Study the drawing (mm; zero at the part's minimum x, y, z) and answer. A direction names the side the tool comes from. Give positions to 0.01 mm unless a question says otherwise; leave off trailing zeros. Order: outer loops, then holes, each group sorted by start corner. A loop starts at its lowest first (then second) coordinate and runs counter-clockwise, first axis right, second up. Notation, with made-up numbers: (-11.75, -37) - (-6.75, -37) arc R23 ccw to (-6.75, -13) - close; hole circle Ø5 at (76, 15). An arc over 180 degrees is marked (long way). Return JSON: item names as keys, results as strings.
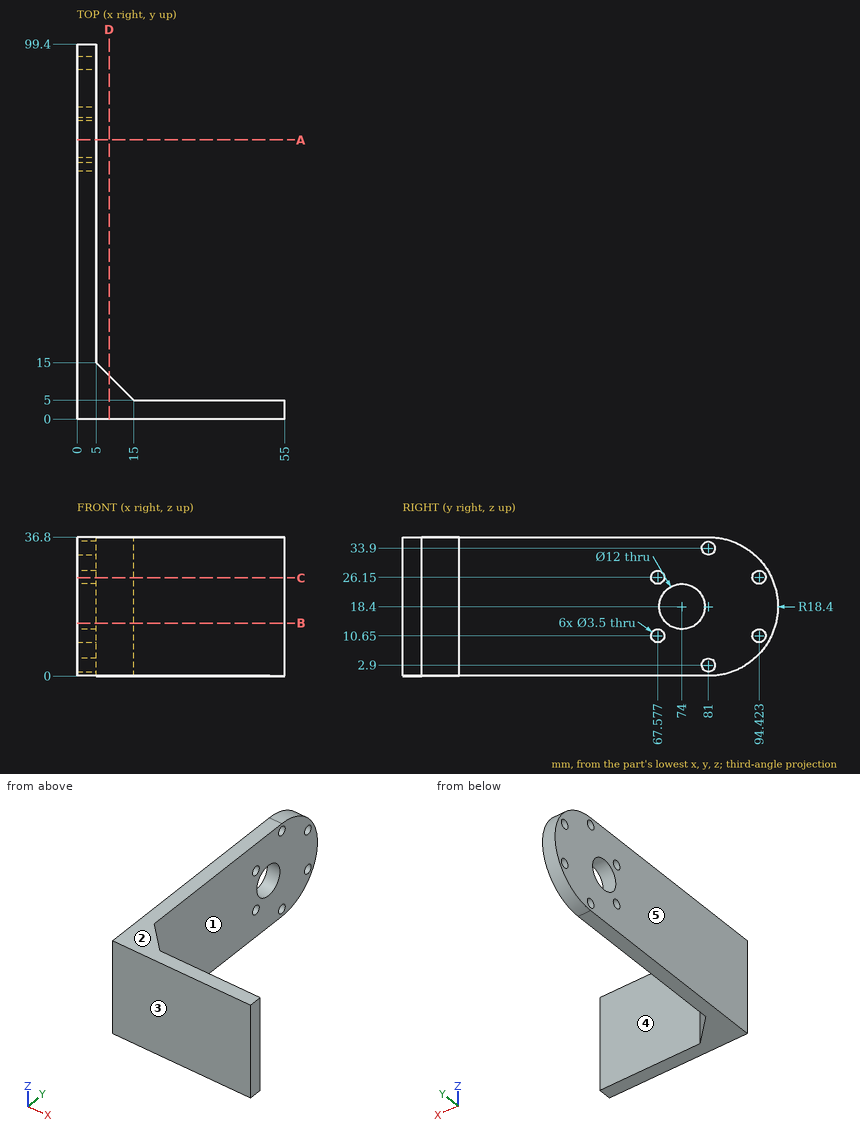
Q1. For the marked faces 1 and 2, determine the directions among +Z, -Z, +X, -X, +Y, -Y from which every point of the face is accessible in a straight line to the end or side of a thin tool.
Values:
{"face 1": "+Z, -Z, +X, +Y", "face 2": "+Z, +X, -X, +Y, -Y"}
Q2. A cutting plane is placed at D-D (x = 8.5). Write down the section's boundary in (y, z).
Values:
{"outline": "(0, 0) - (11.5, 0) - (11.5, 36.8) - (0, 36.8) - close"}
Q3. Determine the mould class of the marked faces 3, 4 and 5 for opening direction Y: released by +Y, released by -Y, zero draft, split by the parting line, or undercut.
Values:
{"face 3": "released by -Y", "face 4": "released by +Y", "face 5": "zero draft"}
Q4. A cutting plane is placed at C-C (z = 26). Write down the section's boundary in (x, y), and give its area (3 significant figures).
Values:
{"outline": "(0, 0) - (55, 0) - (55, 5) - (15, 5) - (5, 15) - (5, 65.83) - (0, 65.83) - close; (0, 69.32) - (5, 69.32) - (5, 92.68) - (0, 92.68) - close; (0, 96.17) - (5, 96.17) - (5, 97.76) - (0, 97.76) - close", "area": "754 mm²"}
Q5. Consider L1, parallel to Z at x = 2, y = 81; L2, parallel to Y at x = 1.1, z = 18.4; L3, parallel to Y at x = 3, z = 10. Determine where each line is inside the solid, lowest interval first.
Values:
{"L1": "z = 0 to 1.15, 4.65 to 32.15, 35.65 to 36.8", "L2": "y = 0 to 68, 80 to 99.4", "L3": "y = 0 to 65.95, 69.2 to 92.8, 96.05 to 97.37"}
Q6. Given pin 1 (3 mm diameter, centred on y = 81, z = 2.9, fed in from -X); pin 2 (6 mm diameter, centred on y = 19.5, z = 29.5, fed in from +X); pin 3 (6 mm diameter, centred on x = 25.5, z = 33, fed in from +Y), each flat-ended and moving along its own axis, determine where each tip first touches the part or whether it passes through.
Values:
{"pin 1": "passes through", "pin 2": "stops at x = 5", "pin 3": "stops at y = 5"}
Q7. A cutting plane is placed at A-A (y = 74). Write down the section's boundary in (x, z), and give its area (3 significant figures).
Values:
{"outline": "(0, 0) - (5, 0) - (5, 12.4) - (0, 12.4) - close; (0, 24.4) - (5, 24.4) - (5, 36.8) - (0, 36.8) - close", "area": "124 mm²"}
Q8. A cutting plane is placed at B-B (z = 14). Write down the section's boundary in (x, y).
Values:
{"outline": "(0, 0) - (55, 0) - (55, 5) - (15, 5) - (5, 15) - (5, 69.92) - (0, 69.92) - close; (0, 78.08) - (5, 78.08) - (5, 98.87) - (0, 98.87) - close"}
